Input: part model. Units: mm. Frame: model coordinates. Give positions to 0.01 mm unless a question says otherwise; leave off trailing zeros. Write each loop counter-clockwise with the first axis right and the second up, starting at its lowest first coordinate (ties: lowest second). Pieces come first, ordered by that corner, then holes.
```python
from build123d import *

# Parameters (mm, degrees)
SKETCH1_R           = 63.5
SKETCH1_R_2         = 50.8
BOSS_EXTRUDE1_DEPTH = 25.4
SKETCH2_W           = 45.380209112
SKETCH2_H           = 34.63225072
CUT_REVOLVE1_ANGLE  = 0.08
SKETCH2_2_W         = 45.380209112
SKETCH2_2_H         = 34.63225072
CUT_REVOLVE2_ANGLE  = 327.2


with BuildPart() as part:
    # Sketch1 → Boss-Extrude1 (new body)
    with BuildSketch(Plane.XY):
        Circle(SKETCH1_R)
        Circle(SKETCH1_R_2, mode=Mode.SUBTRACT)
    extrude(amount=BOSS_EXTRUDE1_DEPTH)

    # Sketch2 → Cut-Revolve1 (revolve, cut)
    with BuildSketch(Plane(origin=(0, 0, 0), x_dir=(1, 0, 0), z_dir=(0, 1, 0))):
        with Locations((-63.5, -12.7)):
            Rectangle(SKETCH2_W, SKETCH2_H)
    revolve(axis=Axis((0, 0, 25.4), (0, 0, -1)), revolution_arc=CUT_REVOLVE1_ANGLE, mode=Mode.SUBTRACT)

    # Sketch2<2> → Cut-Revolve2 (revolve, cut)
    with BuildSketch(Plane(origin=(0, 0, 0), x_dir=(1, 0, 0), z_dir=(0, 1, 0))):
        with Locations((-63.5, -12.7)):
            Rectangle(SKETCH2_2_W, SKETCH2_2_H)
    revolve(axis=Axis((0, 0, 25.4), (0, 0, 1)), revolution_arc=CUT_REVOLVE2_ANGLE, mode=Mode.SUBTRACT)


solid = part.part
```
Item 1: Pin query (flat end, axial travel): pin 1 (1 mm diameter, centred on x = -59.5, z = 18.5, fed in from -Y); pin 2 (2 mm diameter, centred on x = -57.5, y = 12, fed in from -Z); pin 3 (1 mm diameter, centred on x = -46.5, z = 4.5, fed in from +Y); pin 4 (5 mm diameter, centred on y = 23.5, z = 22, fed in from +X). Return the tip coordinate at first contact, or that it passes through.
Item 2: Section A-A (z = 22.5). Return loops of the section in (x, y), and give its area (3 significant figures).
Item 3: Section B-B (x = -54). Return loops of the section in (y, z).
Item 4: Ray query, line 1 (Y direction, x = -58.75, z = 8.5); line 2 (Y direction, x = -43.75, z = 18.75); line 3 (X direction, y = 4, z = 1). Return the intervals inside material, ascending.
Solved:
1. pin 1: stops at y = 0.08
1. pin 2: stops at z = 0
1. pin 3: stops at y = 30.29
1. pin 4: stops at x = -43.64
2. outline: (-63.5, 0.09) - (-50.8, 0.07) arc R50.8 cw to (-42.7, 27.52) - (-53.38, 34.4) arc R63.5 ccw to start
2. area: 414 mm2
3. outline: (0.08, 0) - (33.41, 0) - (33.41, 25.4) - (0.08, 25.4) - close
4. line 1: y = 0.08 to 24.1
4. line 2: y = 25.82 to 28.19
4. line 3: x = -63.37 to -50.64
